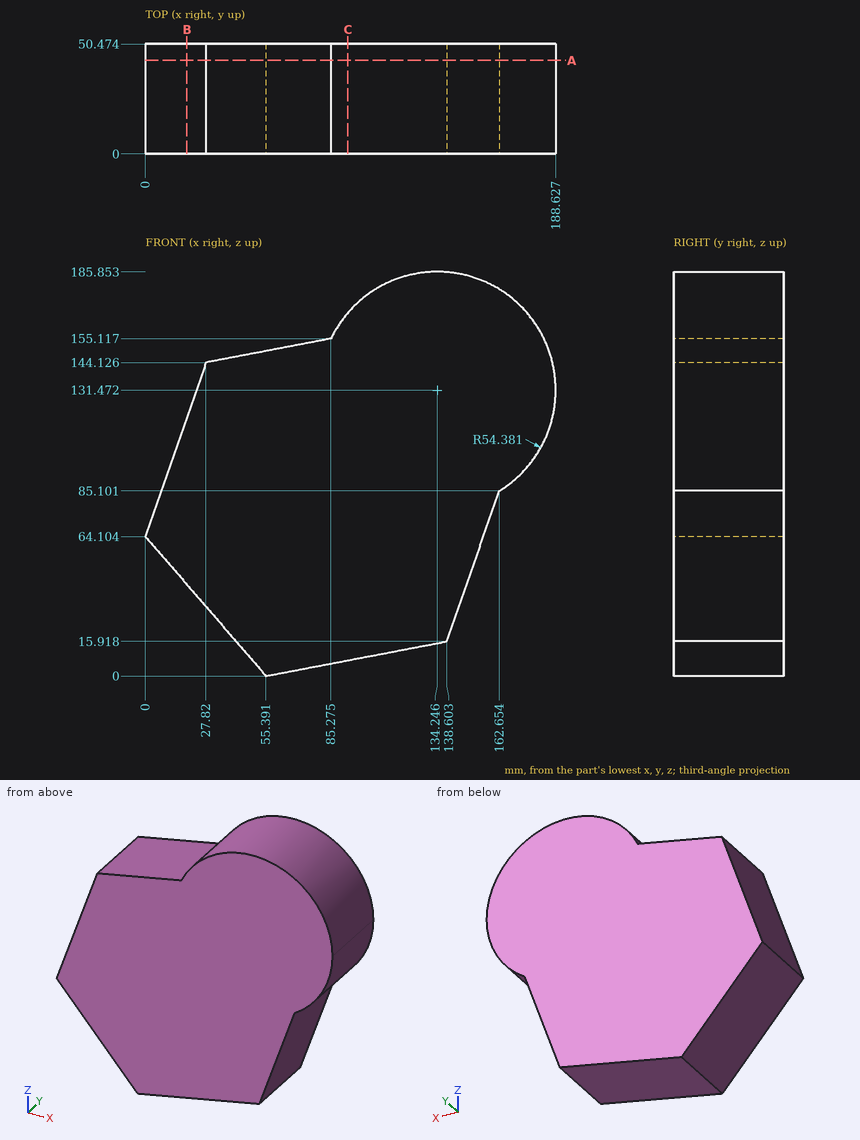
Could you check a few things on this drawing? It's one solid part, dimensions in mm from its lowest x, y, z. Round coordinates to 2 decimals unless told otherwise and drop trailing zeros. Order: outer loops, then holes, each group sorted by start corner. A loop starts at its lowest first (then second) coordinate and runs counter-clockwise, first axis right, second up.
(1) Please list where these lines run through material, in increasing order: line 1 along X through (y, z) = (43.5, 100) (1 decimal); line 2 along Z through (x, y) = (88, 20) (1 decimal); line 3 along Z through (x, y) = (31.5, 27).
Response values:
line 1: x = 12.5 to 178.6
line 2: z = 6.2 to 160.1
line 3: z = 27.65 to 144.83
(2) Imagine slicing it at A-A (y = 43). Write out the boundary of the cut face in (x, z) (1 decimal), plus the area to 3 significant figures.
Response values:
outline: (0, 64.1) - (55.4, 0) - (138.6, 15.9) - (162.7, 85.1) arc R54.4 ccw (long way) to (85.3, 155.1) - (27.8, 144.1) - close
area: 23,400 mm2
(3) I'm going to push flat-ended pins straight in: pin 1 (8 mm diameter, centred on x = 111, y = 28.5, fed in from -Z); pin 2 (1.5 mm diameter, centred on x = 129.5, y = 20, fed in from +Z); pin 3 (2 mm diameter, centred on y = 40, z = 70.5, fed in from +X). Where does each tip first touch, or does it pass through?
Response values:
pin 1: stops at z = 9.87
pin 2: stops at z = 185.71
pin 3: stops at x = 157.93
(4) Imagine slicing it at C-C (x = 93). Write out the boundary of the cut face in (y, z) (1 decimal).
Response values:
outline: (0, 7.2) - (50.5, 7.2) - (50.5, 166.9) - (0, 166.9) - close
(5) Imagine slicing it at B-B (x = 19). Write out the boundary of the cut face in (y, z) (1 decimal).
Response values:
outline: (0, 42.1) - (50.5, 42.1) - (50.5, 118.8) - (0, 118.8) - close
